Could you check a few things on this model? Use its own coordinates, in mm. Face numbers are marked on the shaded views. A direction names the side the tool comes from. Coordinates: 2 decimals unless noted, no trailing zeros. Loops run counter-clockwise (first coordinate to the right, second up) from the corner with the lowest first, then second, coordinate; pieces in that order, holes last.
1) Imagine slicing it at D-D on z = -30. Please give me the cut outline in (x, y).
2) For the marked faces 1 and 2, which set-ups out of +Z, -Z, +X, -X, +Y, -Y let a thin tool reach every point of the face, with its end or its side?
3) Imagine slicing it at B-B on x = -8.5. Please give me the cut outline in (y, z), plus the area to 3 significant figures.
4) Thinking about a two-plate mould opening in Z: for the marked faces 3, 4 and 5, which applies, released by +Z, released by -Z, zero draft, split by the parting line, or undercut?
5) If I drill on line 1 along Z through (x, y) = (9.5, -3); line 2 along X through (y, z) = (3, -39); line 3 along X through (y, z) = (2, -9), over which ranges is the centre line in solid material (lowest first)?
6) Imagine slicing it at C-C on y = 1. Please give me the cut outline in (x, z).
7) Will these pins go through, and if not, where does the flat tip stop? P1, Ø3.5, axis at y = -1, z = -13.5, coming from the +X side; P2, Ø3, axis at y = 2.5, z = -15, coming from the +X side; P3, Ø3.5, axis at x = -22, y = -0.5, coming from the +Z side.
8) Imagine slicing it at A-A on z = -41.5. Please give me the cut outline in (x, y).
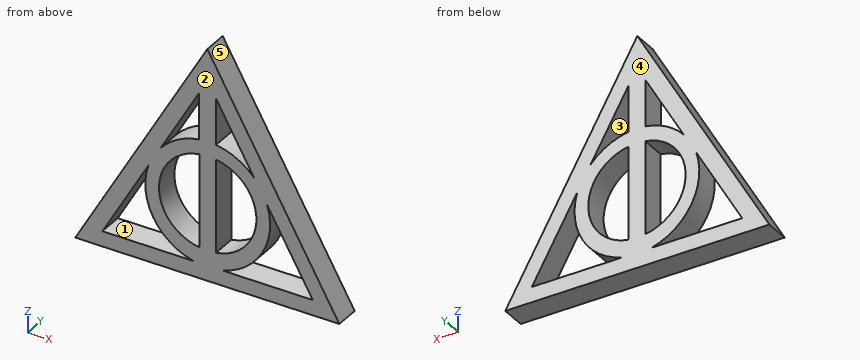
```python
from build123d import *

# Parameters (mm, degrees)
F1_DEPTH = 3.4671
F3_DEPTH = 3.4671


with BuildPart() as f1:
    # F0 (on Front) → F1 (new body, symmetric)
    with BuildSketch(Plane.XZ):
        with BuildLine():
            ThreePointArc((-6.109759, -54.209232), (-2.337391, -54.560416), (1.434976, -54.209232))
            ThreePointArc((1.434976, -54.209232), (15.105103, -36.31727), (0, -19.61905))
            ThreePointArc((0, -19.61905), (-2.337391, -19.35588), (-4.674783, -19.61905))
            ThreePointArc((-4.674783, -19.61905), (-19.779886, -36.31727), (-6.109759, -54.209232))
        make_face()
        with BuildLine():
            ThreePointArc((-4.674783, -49.768269), (-15.959539, -36.759722), (-4.674783, -23.751175))
            Line((-4.674783, -23.751175), (-4.674783, -49.768269))
        make_face(mode=Mode.SUBTRACT)
        with BuildLine():
            ThreePointArc((0, -23.751175), (11.284756, -36.759722), (0, -49.768269))
            Line((0, -49.768269), (0, -23.751175))
        make_face(mode=Mode.SUBTRACT)
    extrude(amount=F1_DEPTH, both=True)

    # F2 (on Front) → F3 (join, symmetric)
    with BuildSketch(Plane.XZ):
        Polygon((34.482322, -58.411262), (-2.444447, 6.384362), (-39.371216, -58.411262), align=None)
        with BuildLine():
            Line((0, -19.747701), (0, -6.65056))
            Line((0, -6.65056), (27.065229, -54.14208))
            Line((27.065229, -54.14208), (-31.788915, -54.14208))
            Line((-31.788915, -54.14208), (-4.723686, -6.65056))
            Line((-4.723686, -6.65056), (-4.723686, -19.747701))
            ThreePointArc((-4.723686, -19.747701), (-2.361843, -19.393884), (0, -19.747701))
        make_face(mode=Mode.SUBTRACT)
    extrude(amount=F3_DEPTH, both=True)


solid = f1.part
```
Filled in:
1. outline: (-23.18, -3.47) - (-14.09, -3.47) - (-14.09, 3.47) - (-23.18, 3.47) - close; (-4.67, -3.47) - (0, -3.47) - (0, 3.47) - (-4.67, 3.47) - close; (9.41, -3.47) - (18.29, -3.47) - (18.29, 3.47) - (9.41, 3.47) - close
2. face 1: +Y, -Y
2. face 2: +Z, -Z, +X, -X, -Y
3. outline: (-3.47, -58.41) - (3.47, -58.41) - (3.47, -54.14) - (-3.47, -54.14) - close; (-3.47, -53.48) - (3.47, -53.48) - (3.47, -48.61) - (-3.47, -48.61) - close; (-3.47, -24.91) - (3.47, -24.91) - (3.47, -20.61) - (-3.47, -20.61) - close; (-3.47, -13.28) - (3.47, -13.28) - (3.47, -4.24) - (-3.47, -4.24) - close
3. area: 156 mm2
4. face 3: undercut
4. face 4: zero draft
4. face 5: released by +Z
5. line 1: z = -58.41 to -54.14, -49.94 to -43.37, -30.15 to -24.15, -23.32 to -14.57
5. line 2: x = -28.31 to -23.16, -19.69 to -15.77, -4.67 to 0, 11.09 to 15.01, 18.44 to 23.42
5. line 3: x = -11.21 to -6.06, -4.72 to 0, 1.34 to 6.32
6. outline: (-39.37, -58.41) - (34.48, -58.41) - (-2.44, 6.38) - close; hole (-31.79, -54.14) - (-6.39, -54.14) arc R17.6 cw to (-18.92, -31.55) - close; hole (-15.44, -25.46) arc R17.6 cw to (-4.72, -19.63) - (-4.72, -6.65) - close; hole (-4.67, -49.77) - (-4.67, -23.75) arc R13.14 ccw to start; hole (0, -49.77) arc R13.14 ccw to (0, -23.75) - close; hole (0, -19.62) arc R17.6 cw to (10.63, -25.3) - (0, -6.65) - close; hole (1.72, -54.14) - (27.07, -54.14) - (14.3, -31.75) arc R17.6 cw to start
7. P1: stops at x = 9.88
7. P2: stops at x = 10.6
7. P3: stops at z = -24.86
8. outline: (-29.73, -3.47) - (-24.58, -3.47) - (-24.58, 3.47) - (-29.73, 3.47) - close; (-19.22, -3.47) - (-15.07, -3.47) - (-15.07, 3.47) - (-19.22, 3.47) - close; (-4.67, -3.47) - (0, -3.47) - (0, 3.47) - (-4.67, 3.47) - close; (10.4, -3.47) - (14.55, -3.47) - (14.55, 3.47) - (10.4, 3.47) - close; (19.86, -3.47) - (24.84, -3.47) - (24.84, 3.47) - (19.86, 3.47) - close
